Verification items for the finished model (mm, model axes). Face numbers are marked on the shaded views. Coordinates: 2 decimals unless noted, no trailing zeros. Loops run counter-clockwise (first coordinate to the right, second up) from the corner with the lowest first, then second, coordinate; pieces in that order, holes last. Notation, with made-up numbers: (60, -39) -> (95, -39) arc R23 cw to (95, -3) -> close; hole circle Ø9 at (-12.5, 24.25). An arc over 180 degrees is marked (long way). Answer as a JSON object with one key per item and string values. Group by question number.
Q1. Cross-section at C-C on z = 2.3. Record the boundary of the cut face in (x, y).
Q2. Release check for a two-part mould opening along X. For the marked faces 1 and 2 record: released by +X, released by -X, zero draft, split by the parting line, or undercut.
Q3. Cross-section at A-A on x = 0. Record the boundary of the cut face in (y, z), and give its area (3 significant figures).
Q4. Gauge pin test, flat ends, axial feed: pin 1 Ø1 at (x, y) = (22, 1) entering from +Z; pin 2 Ø1 at (x, z) = (6, 1) entering from +Y; pin 3 Ø1 at (x, z) = (-27, 2) entering from +Y. Record the tip position at first contact, or that the pin passes through.
Q5. Cross-section at D-D on x = 26.5. Record the boundary of the cut face in (y, z).
Q6. Scan lines: L1, parallel to Y at x = 0, z = 1.75; L2, parallel to X at y = -31, z = 2.8. Record each from-to range of solid material in increasing order.
```python
from build123d import *

# Parameters (mm, degrees)
F0_R     = 38
F2_DEPTH = 1
F1_R     = 39
F1_R_2   = 38
F3_DEPTH = 3
F5_DEPTH = 1


with BuildPart() as f2:
    # F0 (on Top) → F2 (new body)
    with BuildSketch(Plane.XY):
        Circle(F0_R)
    extrude(amount=F2_DEPTH)

    # F1 (on face) → F3 (join)
    with BuildSketch(Plane.XY):
        Circle(F1_R)
        Circle(F1_R_2, mode=Mode.SUBTRACT)
    extrude(amount=F3_DEPTH)

    # F4 (on face) → F5 (join)
    with BuildSketch(Plane.XY):
        with BuildLine():
            ThreePointArc((34.987762, 14.827558), (39.228789, 18.517583), (40.808919, 23.91256))
            ThreePointArc((40.808919, 23.91256), (34.152493, 33.337024), (23.044816, 30.214838))
            ThreePointArc((23.044816, 30.214838), (30.018946, 23.299418), (34.987762, 14.827558))
        make_face()
    extrude(amount=F5_DEPTH)


solid = f2.part
```
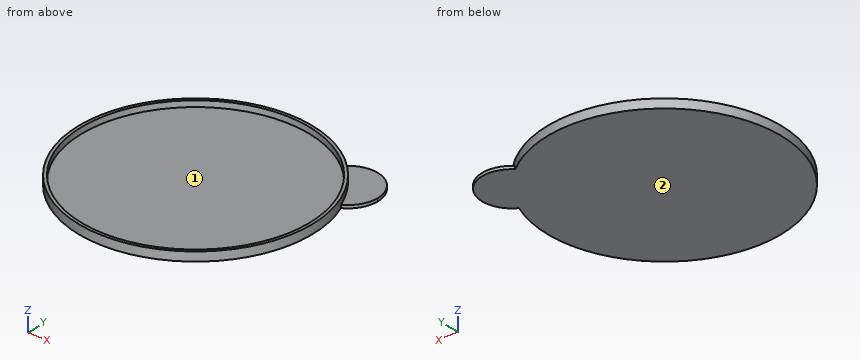
Computed values:
{
 "1": {"outline": "circle Ø78 at (0, 0); hole circle Ø76 at (0, 0)"},
 "2": {"face 1": "undercut", "face 2": "zero draft"},
 "3": {"outline": "(-39, 0) -> (39, 0) -> (39, 3) -> (38, 3) -> (38, 1) -> (-38, 1) -> (-38, 3) -> (-39, 3) -> close", "area": "82.0 mm²"},
 "4": {"pin 1": "stops at z = 1", "pin 2": "stops at y = 38.61", "pin 3": "stops at y = 28.61"},
 "5": {"outline": "(-28.61, 0) -> (32.94, 0) -> (32.94, 1) -> (28.61, 1) -> (28.61, 3) -> (27.24, 3) -> (27.24, 1) -> (-27.24, 1) -> (-27.24, 3) -> (-28.61, 3) -> close"},
 "6": {"L1": "y = -39 to -38, 38 to 39", "L2": "x = -23.66 to -21.98, 21.98 to 23.66"}
}
